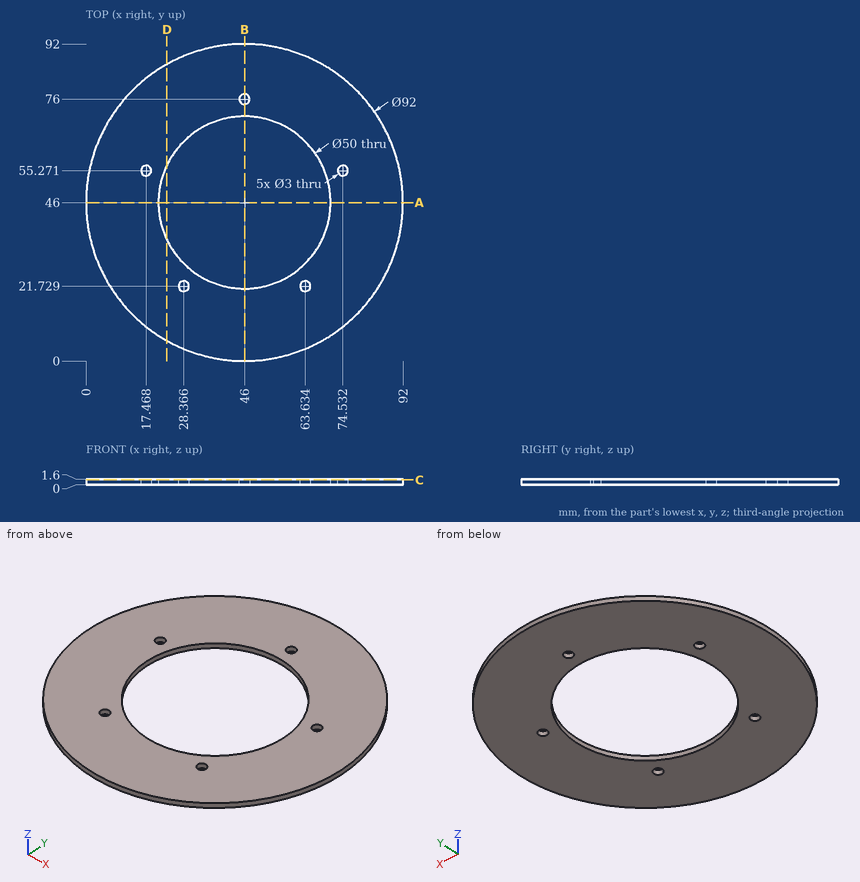
Job drawing, mm, ordinate dimensions from the low corner. One solid piece. Round coordinates to 2 decimals unless told otherwise and drop trailing zeros. Write each loop counter-clockwise with the first axis right and the second up, starting at its lowest first coordinate (ties: lowest second). Pieces come first, ordered by that corner, then holes. Notation, with made-up numbers: M 60.25,87.5 L 94.25,87.5 A16 cw 94.25,100.5 Z; hole C 36.25,38.5 d6. An arc over 180 degrees is marked long. Return JSON: item names as keys, results as strings. Group by question number.
(1) Drill centre lines: probe 1 along Y at (x, z) = (64.5, 0.15) (1 decimal); probe 2 along Y at (x, z) = (46.5, 1.15) (1 decimal); probe 3 along X at (y, z) = (77, 0.6) (1 decimal). Where is each one in solid material? Low to high.
(2) Saw through at B-B on x = 46. Write the cut outline in (y, z).
(3) Saw through at C-C on z = 1.35. Write the cut outline in (x, y), then the cut area to 3 significant figures.
(4) Saw through at A-A on y = 46. Write the cut outline in (x, z).
(5) Saw through at D-D on x = 23.5. Write the cut outline in (y, z).
Returned:
{
 "1": {"probe 1": "3.9 to 20.5, 23 to 29.2, 62.8 to 88.1", "probe 2": "0 to 21, 71 to 74.6, 77.4 to 92", "probe 3": "12 to 44.9, 47.1 to 80"},
 "2": {"outline": "M 0,0 L 21,0 L 21,1.6 L 0,1.6 Z; M 71,0 L 74.5,0 L 74.5,1.6 L 71,1.6 Z; M 77.5,0 L 92,0 L 92,1.6 L 77.5,1.6 Z"},
 "3": {"outline": "C 46,46 d92; hole C 17.47,55.27 d3; hole C 46,46 d50; hole C 28.37,21.73 d3; hole C 46,76 d3; hole C 63.63,21.73 d3; hole C 74.53,55.27 d3", "area": "4,650 mm²"},
 "4": {"outline": "M 0,0 L 21,0 L 21,1.6 L 0,1.6 Z; M 71,0 L 92,0 L 92,1.6 L 71,1.6 Z"},
 "5": {"outline": "M 5.88,0 L 35.1,0 L 35.1,1.6 L 5.88,1.6 Z; M 56.9,0 L 86.12,0 L 86.12,1.6 L 56.9,1.6 Z"}
}
